Autodesk Inventor part; units mm, degrees
ref_plane "YZ Plane" through (0, 0, 0) normal (1, 0, 0) x (0, 1, 0)
ref_plane "XZ Plane" through (0, 0, 0) normal (0, 1, 0) x (-1, 0, 0)
ref_plane "XY Plane" through (0, 0, 0) normal (0, 0, 1) x (1, 0, 0)
sketch "Sketch1" plane through (0, 0, 0) normal (0, 0, 1) x (1, 0, 0)
  circle A0 centre (0, 0) radius 9.7536
  line L0 (-7.3323, 0) -> (-3.6662, 6.35)
  line L1 (-3.6662, 6.35) -> (3.6662, 6.35)
  line L2 (3.6662, 6.35) -> (7.3323, 0)
  line L3 (7.3323, 0) -> (3.6662, -6.35)
  line L4 (3.6662, -6.35) -> (-3.6662, -6.35)
  line L5 (-3.6662, -6.35) -> (-7.3323, 0)
  dimension "d0" = 19.5072
  dimension "d1" = 12.7
extrude "Extrusion1" add sketch "Sketch1" along normal blind 1.5875
properties part number "acetalspacer" material "PVC-Piping"
Verification items for the finished model (mm, model axes). A direction names the side the tool comes from. Give positions to 0.01 mm unless a question says otherwise; leave off trailing zeros. Write each loop counter-clockwise with the first axis right and the second up, starting at its lowest first coordinate (ties: lowest second). Pieces come first, ordered by that corner, then holes. Notation, with made-up numbers: M 29,34 L 46,34 A20 ccw 46,51 Z; hole C -0.75,52 d8. An arc over 180 degrees is marked long. Write item = value, one per line.
(1) Access from +Z, -Z, +X, -X, +Y, -Y to the whole of each face (thin tool, end or side, straight path). Record for faces 4 (the face through (6.4, -2, 0)), 5 (the face through (-5.525, 3.131, 0.783)).
Found:
face_4 = -Z, +X, -X, +Y, -Y
face_5 = +Z, -Z
(2) Sectioned sample at A-A (z = 0.8). Record the cut outline in (x, y).
Found:
outline = C 0,0 d19.51; hole M -7.33,0 L -3.67,-6.35 L 3.67,-6.35 L 7.33,0 L 3.67,6.35 L -3.67,6.35 Z
(3) Draft check along Y on faces 1 (the face through (-5.474, -3.219, 0.783)), 2 (the face through (6.4, -2, 1.588)), 3 (the face through (9.303, -2.93, 0.783)). Enter one of: released by +Y, released by -Y, zero draft, split by the parting line, or undercut.
Found:
face_1 = undercut
face_2 = zero draft
face_3 = split by the parting line
(4) Sectioned sample at B-B (x = 0). Record the cut outline in (y, z).
Found:
outline = M -9.75,0 L -6.35,0 L -6.35,1.59 L -9.75,1.59 Z; M 6.35,0 L 9.75,0 L 9.75,1.59 L 6.35,1.59 Z
(5) Sectioned sample at D-D (x = 8.5). Record the cut outline in (y, z).
Found:
outline = M -4.78,0 L 4.78,0 L 4.78,1.59 L -4.78,1.59 Z
(6) Material ranges on line 1 (Y direction, x = -0.25, z = 0.55); line 2 (Y direction, x = -3, z = 0.8); line 3 (X direction, y = 2.25, z = 0.2), recorded low to high.
Found:
line_1 = -9.75 to -6.35, 6.35 to 9.75
line_2 = -9.28 to -6.35, 6.35 to 9.28
line_3 = -9.49 to -6.03, 6.03 to 9.49
(7) Go/stop test with a flat-tipped pin: pin 1 Ø0.5 at (x, z) = (-1, 0.5) entering from +Y. Record where the tip stops, or that it passes through.
Found:
pin_1 = 9.72
(8) Sectioned sample at C-C (y = -5). Record the cut outline in (x, z), then the cut area to 3 significant figures.
Found:
outline = M -8.37,0 L -4.45,0 L -4.45,1.59 L -8.37,1.59 Z; M 4.45,0 L 8.37,0 L 8.37,1.59 L 4.45,1.59 Z
area = 12.5 mm2
